Check sheet for the modelled part. Datum: model origin and axes. Units: mm. A direction names the side the tool comes from. Coordinates: 2 decimals unless noted, no trailing zeros. Loops run counter-clockwise (first coordinate to the right, second up) from the corner with the lowest first, then second, coordinate; pieces in that order, holes last. Notation, with made-up numbers: M 45,-4 L 71,-4 A21 ccw 71,11 Z; hole C 15.25,76 d4. An arc over 180 degrees is marked long. Answer in a Markdown table with one row per item. Add a question column.
```python
from build123d import *

# Parameters (mm, degrees)
SKETCH1_R                = 100.0125
SKETCH1_R_2              = 95.25
EXTRUDE_THIN1_DEPTH      = 165.1
BOSS_EXTRUDE1_DEPTH      = 6.35
FILLET1_R                = 3.302
CIRPATTERN1_COUNT        = 3
FILLET1_OF_CIRPATTERN1_R = 3.302
MIRROR2_START            = -165.1
MIRROR2_DEPTH            = 6.35


# Read off the part's stored shape, not the designer's step: Mirror2
with BuildPart() as part:
    # Sketch1 → Extrude-Thin1 (new, symmetric)
    with BuildSketch(Plane.XY):
        Circle(SKETCH1_R)
        Circle(SKETCH1_R_2, mode=Mode.SUBTRACT)
    extrude(amount=EXTRUDE_THIN1_DEPTH, both=True)

    # Sketch2 → Boss-Extrude1 (add)
    with BuildSketch(Plane.XY.offset(165.1)):
        with BuildLine():
            ThreePointArc((-12.674375762, 99.206150794), (0, 112.7125), (12.674375762, 99.206150794))
            ThreePointArc((12.674375762, 99.206150794), (0, 100.0125), (-12.674375762, 99.206150794))
        make_face()
    boss_extrude1 = extrude(amount=-BOSS_EXTRUDE1_DEPTH)

    # Fillet1
    fillet1_edges = [part.edges().sort_by_distance(p)[0] for p in [
        (12.674375762, 99.206150794, 161.925),
        (-12.674375762, 99.206150794, 161.925),
    ]]
    fillet(fillet1_edges, radius=FILLET1_R)

    # CirPattern1: Boss-Extrude1 ×3 about axis
    cirpattern1_axis = Axis((0, 0, 0), (0, 0, 1))
    for i in range(1, CIRPATTERN1_COUNT):
        add(boss_extrude1.rotate(cirpattern1_axis, i * 360 / CIRPATTERN1_COUNT))

    # Fillet1 of CirPattern1
    fillet1_of_cirpattern1_edges = [part.edges().sort_by_distance(p)[0] for p in [
        (-92.25223468, -38.62674401, 161.925),
        (-79.577858918, -60.579406784, 161.925),
        (79.577858918, -60.579406784, 161.925),
        (92.25223468, -38.62674401, 161.925),
    ]]
    fillet(fillet1_of_cirpattern1_edges, radius=FILLET1_OF_CIRPATTERN1_R)

    # Mirror2 outline → Mirror2 (add)
    with BuildSketch(Plane.XY.offset(MIRROR2_START)):
        with BuildLine():
            ThreePointArc((12.592634281, 101.660396196), (0, 112.7125), (-12.592634281, 101.660396196))
            ThreePointArc((-12.592634281, 101.660396196), (-13.503928486, 99.78224476), (-15.359608316, 98.826021819))
            ThreePointArc((-15.359608316, 98.826021819), (0, 100.0125), (15.359608316, 98.826021819))
            ThreePointArc((15.359608316, 98.826021819), (13.503928486, 99.78224476), (12.592634281, 101.660396196))
        make_face()
        with BuildLine():
            ThreePointArc((-77.906041293, -62.714821903), (-86.613365696, -50.00625), (-93.265649608, -36.111199916))
            ThreePointArc((-93.265649608, -36.111199916), (-93.165923052, -38.19637726), (-94.336802804, -39.92465691))
            ThreePointArc((-94.336802804, -39.92465691), (-97.611888324, -56.35625), (-81.744168524, -61.735739285))
            ThreePointArc((-81.744168524, -61.735739285), (-79.661994566, -61.5858675), (-77.906041293, -62.714821903))
        make_face()
        with BuildLine():
            ThreePointArc((94.336802804, -39.92465691), (93.165923052, -38.19637726), (93.265649608, -36.111199916))
            ThreePointArc((93.265649608, -36.111199916), (86.613365696, -50.00625), (77.906041293, -62.714821903))
            ThreePointArc((77.906041293, -62.714821903), (79.661994566, -61.5858675), (81.744168524, -61.735739285))
            ThreePointArc((81.744168524, -61.735739285), (97.611888324, -56.35625), (94.336802804, -39.92465691))
        make_face()
    extrude(amount=MIRROR2_DEPTH)


solid = part.part
```
Q1. Cross-section at D-D (x = -55.5). Record the cut outline in (y, z).
Q2. Thickness scan on L1, parallel to Y at x = 0, z = -34.5; L2, parallel to Z at x = 90, y = -47.5; L3, parallel to Y at x = -33.5, z = -121. Record the ranges inside material, lowest first.
Q3. Cross-section at A-A (x = 0). Record the cut outline in (y, z).
Q4. Mould release check, pull along Y, two halves, no side actions. Record for faces 1 (the face through (92, -53, 158.75)), 2 (the face through (-97.48, -56.58, 161.97)), 3 (the face through (0.26, 112.71, -161.97)): released by +Y, released by -Y, zero draft, split by the parting line, or undercut.
Q5. Go/stop test with flat-tipped pins: pin 1 (1 mm diameter, centred on x = -46, z = -108, fed in from +Y); pin 2 (3 mm diameter, centred on y = 44, z = -85.5, fed in from -X); pin 3 (1.5 mm diameter, centred on x = 7.5, z = -17.5, fed in from +Y). Record where each tip stops, or that it passes through.
Q6. Cross-section at B-B (y = 0). Record the cut outline in (x, z), plus the area to 3 significant figures.
Q7. Access from +Z, -Z, +X, -X, +Y, -Y to the whole of each face (thin tool, end or side, straight path). Record for faces 4 (the face through (-75.587, -57.958, -2.311)), 5 (the face through (91, -52, -158.75)), 6 (the face through (-21.681, -97.634, 2.311)), 7 (the face through (-91, -52, -158.75)), 8 (the face through (0, -96, 165.1)).
Answer key:
| question | item | result |
|---|---|---|
| 1 | outline | M -83.2,-165.1 L -77.41,-165.1 L -77.41,165.1 L -83.2,165.1 Z; M 77.41,-165.1 L 83.2,-165.1 L 83.2,165.1 L 77.41,165.1 Z |
| 2 | L1 | -100.01 to -95.25, 95.25 to 100.01 |
| 2 | L2 | -165.1 to -158.75, 158.75 to 165.1 |
| 2 | L3 | -94.24 to -89.16, 89.16 to 94.24 |
| 3 | outline | M -100.01,-165.1 L -95.25,-165.1 L -95.25,165.1 L -100.01,165.1 Z; M 95.25,-165.1 L 112.71,-165.1 L 112.71,-158.75 L 100.01,-158.75 L 100.01,158.75 L 112.71,158.75 L 112.71,165.1 L 95.25,165.1 Z |
| 4 | face 1 | zero draft |
| 4 | face 2 | undercut |
| 4 | face 3 | released by +Y |
| 5 | pin 1 | y = 89.06 |
| 5 | pin 2 | x = -90.53 |
| 5 | pin 3 | y = 99.78 |
| 6 | outline | M -100.01,-165.1 L -95.25,-165.1 L -95.25,165.1 L -100.01,165.1 Z; M 95.25,-165.1 L 100.01,-165.1 L 100.01,165.1 L 95.25,165.1 Z |
| 6 | area | 3,150 mm^2 |
| 7 | face 4 | +Z, -Z |
| 7 | face 5 | +X, -Y |
| 7 | face 6 | none |
| 7 | face 7 | -X, -Y |
| 7 | face 8 | +Z, +X, -X, +Y, -Y |
